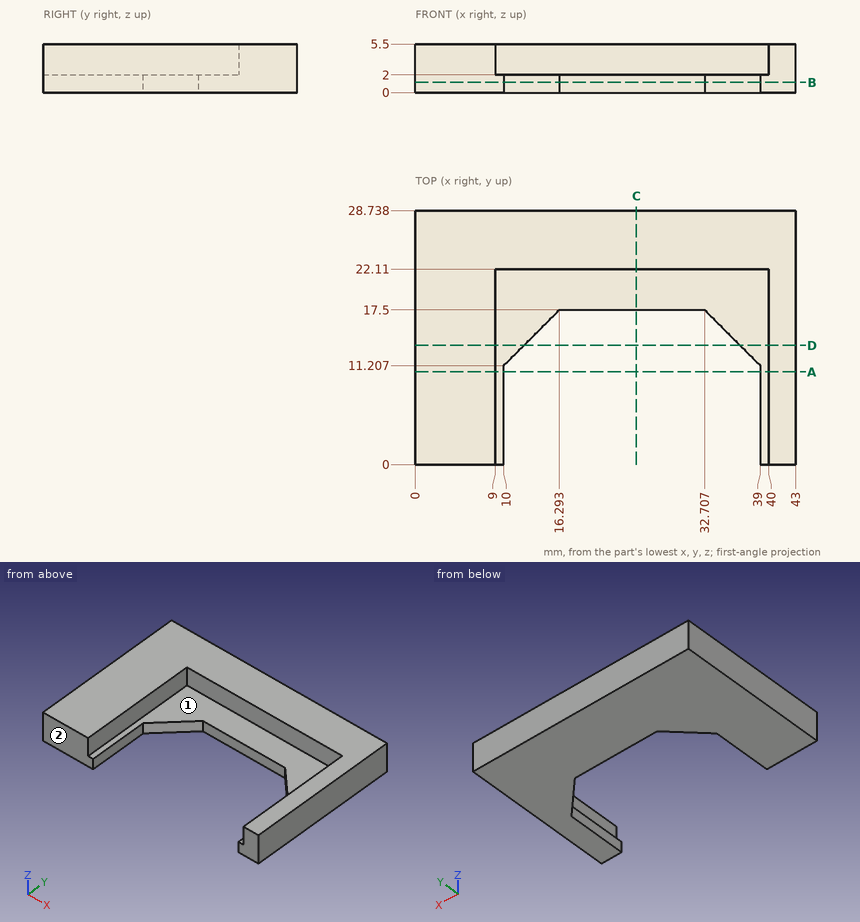
The drawing under review shows one solid part. Ordinate dimensions are in mm from its lowest x, y, z. A direction names the side the tool comes from. Give positions to 0.01 mm unless a question says otherwise; leave off trailing zeros. Order: outer loops, then holes, each group sorted by start corner. A loop starts at its lowest first (then second) coordinate and runs counter-clockwise, first axis right, second up. Notation, with made-up numbers: (11, 87) -> (51, 87) arc R29 cw to (51, 126) -> close; hole circle Ø11 at (81, 63). An arc over 180 degrees is marked (long way). Write item = value, one per line.
1) We need section D-D, the plane y = 13.5. Give the boundary of the cut face in (x, z).
Findings:
outline = (0, 0) -> (12.29, 0) -> (12.29, 2) -> (9, 2) -> (9, 5.5) -> (0, 5.5) -> close; (36.71, 0) -> (43, 0) -> (43, 5.5) -> (40, 5.5) -> (40, 2) -> (36.71, 2) -> close
2) We need section C-C, the plane x = 25. Give the boundary of the cut face in (y, z), and give its area (3 significant figures).
Findings:
outline = (17.5, 0) -> (28.74, 0) -> (28.74, 5.5) -> (22.11, 5.5) -> (22.11, 2) -> (17.5, 2) -> close
area = 45.7 mm^2
3) To check wall thickness, follow L1, parallel to X at y = 5.25, z = 2.15; L2, parallel to Y at x = 20, z = 0.25; L3, parallel to Z at x = 37.5, y = 19.5. State the ranges of each line that lie inside material, in increasing order. Write a range as from..to.
Findings:
L1 = 0..9, 40..43
L2 = 17.5..28.74
L3 = 0..2
4) We need section B-B, the plane z = 1.15. Give the boundary of the cut face in (x, y), and give its area (3 significant figures).
Findings:
outline = (0, 0) -> (10, 0) -> (10, 11.21) -> (16.29, 17.5) -> (32.71, 17.5) -> (39, 11.21) -> (39, 0) -> (43, 0) -> (43, 28.74) -> (0, 28.74) -> close
area = 768 mm^2
5) We need section A-A, the plane y = 10.5. Give the boundary of the cut face in (x, z), and give its area (3 significant figures).
Findings:
outline = (0, 0) -> (10, 0) -> (10, 2) -> (9, 2) -> (9, 5.5) -> (0, 5.5) -> close; (39, 0) -> (43, 0) -> (43, 5.5) -> (40, 5.5) -> (40, 2) -> (39, 2) -> close
area = 70.0 mm^2
6) Insertion check: pin 1 (2 mm diameter, centred on x = 27, z = 0.5, fed in from -Y); pin 2 (1 mm diameter, centred on y = 23.5, z = 3.5, fed in from -X). Each pin has a flat end and moves straight along its axis. Give the tip position at first contact, or say it passes through.
Findings:
pin_1 = 17.5
pin_2 = 0
7) For the marked faces 1 and 2, list the 3-axis set-ups (+Z, -Z, +X, -X, +Y, -Y) from which the entire face can be reached by the end or side of a thin tool; tool diameter is ignored.
Findings:
face_1 = +Z, -Y
face_2 = +Z, -Z, +X, -X, -Y
